```python
from build123d import *

# Parameters (mm, degrees)
F0_W     = 25.4
F0_H     = 31.75
F1_DEPTH = 38.1
F3_DEPTH = 25.4
F4_DEPTH = 25.4
F6_DEPTH = 16.9333333333


# Not quite as in the source:
# - a length typed as a fraction of an inch, garbled in the dataset ("3 / 203.2 mm" for 3/8 in), is restored


with BuildPart() as f1:
    # F0 (on Right) → F1 (new body)
    with BuildSketch(Plane.YZ):
        with Locations((31.233229906, 15.875)):
            Rectangle(F0_W, F0_H)
    extrude(amount=F1_DEPTH)

    # F2 (on Right) → F3 (cut)
    with BuildSketch(Plane.YZ):
        Polygon((43.7832586467, 31.5612442791), (24.7332586467, 31.5612442791), (44.0856164074, 6.1630439534), align=None)
    extrude(amount=-F3_DEPTH, mode=Mode.SUBTRACT)

    # F2 (on Right) → F4 (cut)
    with BuildSketch(Plane.YZ):
        Polygon((43.7832586467, 31.5612442791), (24.7332586467, 31.5612442791), (44.0856164074, 6.1630439534), align=None)
    extrude(amount=-F4_DEPTH, mode=Mode.SUBTRACT)

    # F5 (on face) → F6 (cut)
    with BuildSketch(Plane.YZ.offset(38.1)):
        Polygon((18.533229906, 6.35), (37.583229906, 31.75), (18.533229906, 31.75), align=None)
    extrude(amount=-F6_DEPTH, mode=Mode.SUBTRACT)


solid = f1.part
```
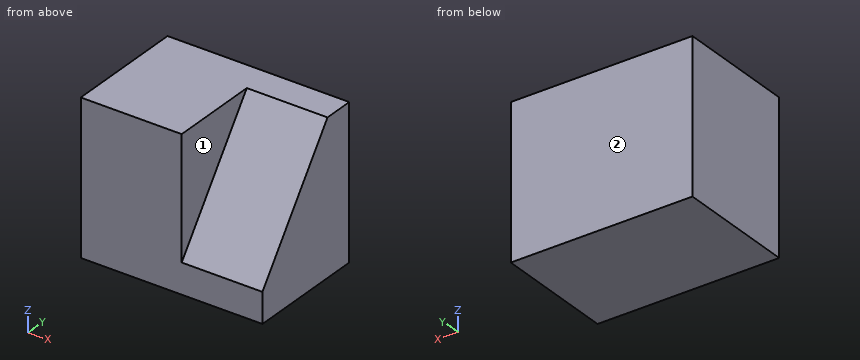
CAD build for the part. Positions are in the model's coordinates, mm. Face numbers are marked on the shaded views. A direction names the side the tool comes from. Round coordinates to 2 decimals unless told otherwise and drop trailing zeros. Write each loop counter-clockwise with the first axis right and the second up, starting at its lowest first coordinate (ties: lowest second). Pieces come first, ordered by that corner, then holes. Notation, with made-up numbers: M 31,37 L 71,37 A21 ccw 71,63 Z; hole C 87,-26 d10. An arc over 180 degrees is marked long. One line per question, with ' | ' between items.
1. Pin check, flat tip, straight feed: pin 1 Ø15 at (y, z) = (24.5, 23) entering from +X. Stop position of the tip, or through.
Working result:
pin 1: x = 38.1
2. Probe L1, parallel to X at y = 26.75, z = 25; L2, parallel to Y at x = 23.5, z = 20.5; L3, parallel to Y at x = 25, z = 19.5. List the from-to ranges inside material, lowest first. Write a range as from..to.
Working result:
L1: 0..21.17 | L2: 29.15..43.93 | L3: 28.4..43.93
3. Cut at C-C on y = 30.5. Write the cut outline in (x, z).
Working result:
outline: M 0,0 L 38.1,0 L 38.1,22.31 L 21.17,22.31 L 21.17,31.75 L 0,31.75 Z
4. Cut at A-A on x = 22. Write the cut outline in (y, z).
Working result:
outline: M 18.53,0 L 43.93,0 L 43.93,31.75 L 37.58,31.75 L 18.53,6.35 Z
5. Which spindle directions (+Z, -Z, +X, -X, +Y, -Y) get a long thin tool onto all of the face, cutting with end or side? Do the marked faces 1 and 2. Say none if no direction does.
Working result:
face 1: +Z, +X, -Y | face 2: +Z, -Z, +X, -X, +Y
6. Cut at B-B on z = 13. Write the cut outline in (x, y), and give its area (3 significant figures).
Working result:
outline: M 0,18.53 L 21.17,18.53 L 21.17,23.52 L 38.1,23.52 L 38.1,43.93 L 0,43.93 Z | area: 883 mm2
